```python
from build123d import *

# Parameters (mm, degrees)
F3_DEPTH = 2.6543
F4_W     = 114.3
F4_H     = 38.1
F5_DEPTH = 2.6543
F6_R     = 10.0457
F7_R     = 12.7
F8_R     = 19.05
F10_D    = 6.7564
F12_D    = 6.7564


with BuildPart() as f3:
    # F2 (on offset) → F3 (new body)
    with BuildSketch(Plane.XZ.offset(19.05)):
        Polygon((57.15, 0), (0, 0), (-57.15, 0), (-57.15, -25.4), (-19.05, -101.6), (0, -101.6), (19.05, -101.6), (57.15, -25.4), align=None)
    extrude(amount=F3_DEPTH)

    # F4 (on face) → F5 (join)
    with BuildSketch(Plane.XY):
        with Locations((0, -38.1)):
            Rectangle(F4_W, F4_H)
    extrude(amount=-F5_DEPTH)

    # F6
    f6_edges = [f3.edges().sort_by_distance(p)[0] for p in [
        (0, -21.7043, -2.6543),
    ]]
    fillet(f6_edges, radius=F6_R)

    # F7
    f7_edges = [f3.edges().sort_by_distance(p)[0] for p in [
        (0, -19.05, 0),
    ]]
    fillet(f7_edges, radius=F7_R)

    # F8
    f8_edges = [f3.edges().sort_by_distance(p)[0] for p in [
        (-57.15, -57.15, -1.32715),
        (57.15, -57.15, -1.32715),
        (-57.15, -20.37715, -25.4),
        (57.15, -20.37715, -25.4),
        (19.05, -20.37715, -101.6),
        (-19.05, -20.37715, -101.6),
    ]]
    fillet(f8_edges, radius=F8_R)

    # F10 (through all)
    with Locations(Plane.XY):
        with Locations((-44.45, -44.45), (44.45, -44.45)):
            Hole(F10_D / 2)

    # F12 (through all)
    with Locations(Plane.XZ.offset(21.7043)):
        with Locations((0, -25.4), (0, -88.9)):
            Hole(F12_D / 2)


solid = f3.part
```
The listing builds one solid part. Answer for the finished solid, in the listing's coordinates (mm). A direction names the side the tool comes from. Round coordinates to 2 decimals unless told otherwise and drop trailing zeros. Loops run counter-clockwise (first coordinate to the right, second up) from the corner with the lowest first, then second, coordinate; pieces in that order, holes last.
Q1. For a pull along X with two mould halves and no side action, classify faces 3 (the face through (-57.15, -24, -6)), 4 (the face through (51.42, -51.72, -1.35)), 5 (the face through (0.73, -20.36, -28.7)) as released by +X, released by -X, zero draft, split by the parting line, or undercut.
Q2. Given pin 1 Ø3 at (x, y) = (-18.5, -24.5) entering from -Z; pin 2 Ø10 at (x, z) = (29.5, -69.5) entering from -Y; pin 3 Ø7.5 at (x, y) = (-26.5, -41) entering from -Z, each flat-ended and moving along its own axis, determine where each tip first touches the part or whether it passes through.
Q3. Section B-B, the plane x = 43 is taken. Determine the outline of the cut face in (y, z).
Q4. Section C-C, the plane y = -44.45 is taken. Determine the outline of the cut face in (x, z).
Q5. Section A-A, the plane z = -88.9 is taken. Determine the outline of the cut face in (x, y), then the cut area to 3 significant figures.
Q6. Which of the six approach directions +Z, -Z, +X, -X, +Y, -Y give full straight-line access (tool end or side, diameter ignored) to faces 1 (the face through (-1.816, -20.359, -86.051)), 2 (the face through (-1, -21.704, -47))?
Q7. Section D-D, the plane z = -25.4 is taken. Determine the outline of the cut face in (x, y).
Q8. Find the intervals of material crossed by line 1 (Z direction, x = 0, y = -20); line 2 (Z direction, x = 0, y = -21); line 3 (Y direction, x = -30.5, z = -36.5), in increasing order.
Completed:
1. face 3: released by -X
1. face 4: released by +X
1. face 5: undercut
2. pin 1: stops at z = -7.77
2. pin 2: stops at y = -21.7
2. pin 3: stops at z = -2.65
3. outline: (-56.51, -2.65) - (-47.5, -2.65) - (-47.5, 0) - (-56.51, 0) - close; (-41.4, -2.65) - (-31.75, -2.65) arc R10.05 cw to (-21.7, -12.7) - (-21.7, -53.7) - (-19.05, -53.7) - (-19.05, -12.7) arc R12.7 ccw to (-31.75, 0) - (-41.4, 0) - close
4. outline: (-56.06, -2.65) - (-47.83, -2.65) - (-47.83, 0) - (-56.06, 0) - close; (-41.07, -2.65) - (41.07, -2.65) - (41.07, 0) - (-41.07, 0) - close; (47.83, -2.65) - (56.06, -2.65) - (56.06, 0) - (47.83, 0) - close
5. outline: (-25.4, -21.7) - (-3.38, -21.7) - (-3.38, -19.05) - (-25.4, -19.05) - close; (3.38, -21.7) - (25.4, -21.7) - (25.4, -19.05) - (3.38, -19.05) - close
5. area: 117 mm2
6. face 1: +Y, -Y
6. face 2: -Z, +X, -X, -Y
7. outline: (-56.61, -21.7) - (-3.38, -21.7) - (-3.38, -19.05) - (-56.61, -19.05) - close; (3.38, -21.7) - (56.61, -21.7) - (56.61, -19.05) - (3.38, -19.05) - close
8. line 1: z = -101.6 to -92.28, -85.52 to -28.78, -22.02 to -7.88
8. line 2: z = -101.6 to -92.28, -85.52 to -28.78, -22.02 to -5.94
8. line 3: y = -21.7 to -19.05
